```python
from build123d import *

# Parameters (mm, degrees)
F1_DEPTH     = 50.8
F3_DEPTH     = 25.4
F4_T1_DEPTH  = 50.8
F4_T6_DEPTH  = 30.48
F4_S7_R      = 7.62
F4_T8_DEPTH  = 17
F4_T12_DEPTH = 30.48
F4_S13_R     = 7.62
F4_T14_DEPTH = 17
F6_D         = 7.62


# Not quite as in the source:
# - a fillet or chamfer that OpenCascade refuses, or shapes differently, is made with other operations: its cross-section is extruded or revolved along the edge and cut away or added


with BuildPart() as f1:
    # F0 (on Top) → F1 (new body)
    with BuildSketch(Plane.XY):
        with BuildLine():
            Line((0, 25.4), (0, 0))
            Line((0, 0), (50.8, 0))
            Line((50.8, 0), (50.8, 5.08))
            ThreePointArc((50.8, 5.08), (43.18, 12.7), (50.8, 20.32))
            Line((50.8, 20.32), (50.8, 25.4))
            Line((50.8, 25.4), (0, 25.4))
        make_face()
        with BuildLine():
            Line((50.8, 20.32), (50.8, 5.08))
            ThreePointArc((50.8, 5.08), (56.1881536726, 7.3118463274), (58.42, 12.7))
            ThreePointArc((58.42, 12.7), (56.1881536726, 18.0881536726), (50.8, 20.32))
        make_face()
        with BuildLine():
            ThreePointArc((50.8, 20.32), (43.18, 12.7), (50.8, 5.08))
            Line((50.8, 5.08), (50.8, 20.32))
        make_face()
    extrude(amount=F1_DEPTH)

    # F2 (on face) → F3 (cut)
    with BuildSketch(Plane.XZ):
        with BuildLine():
            ThreePointArc((38.1, 25.4), (25.4, 38.1), (12.7, 25.4))
            Line((12.7, 25.4), (38.1, 25.4))
        make_face()
        with BuildLine():
            Line((38.1, 25.4), (12.7, 25.4))
            ThreePointArc((12.7, 25.4), (25.4, 12.7), (38.1, 25.4))
        make_face()
        with BuildLine():
            Line((12.7, 25.4), (12.7, 0))
            Line((12.7, 0), (38.1, 0))
            Line((38.1, 0), (38.1, 25.4))
            ThreePointArc((38.1, 25.4), (25.4, 12.7), (12.7, 25.4))
        make_face()
    extrude(amount=-F3_DEPTH, mode=Mode.SUBTRACT)

    # F4: fillet of radius 5.08 on 3 edges, made by hand

    # F4_s2 → F4_t1 (cut)
    with BuildSketch(Plane.XZ.offset(-38.1)):
        with BuildLine():
            ThreePointArc((0, 45.72), (1.4878975516, 49.3121024484), (5.08, 50.8))
            Line((5.08, 50.8), (0, 50.8))
            Line((0, 50.8), (0, 45.72))
        make_face()
    extrude(amount=F4_T1_DEPTH, mode=Mode.SUBTRACT)


with BuildPart() as f4_tool4:
    # F4_s5 → F4_t6 (new body)
    with BuildSketch(Plane.XZ.offset(12.7)):
        with BuildLine():
            ThreePointArc((45.72, 50.8), (49.3121024484, 49.3121024484), (50.8, 45.72))
            Line((50.8, 45.72), (50.8, 50.8))
            Line((50.8, 50.8), (45.72, 50.8))
        make_face()
    extrude(amount=-F4_T6_DEPTH)

    # F4_s7 → F4_t8 (cut, symmetric)
    with BuildSketch(Plane.XY.offset(48.3)):
        with Locations((50.8, 12.7)):
            Circle(F4_S7_R)
    extrude(amount=F4_T8_DEPTH, both=True, mode=Mode.SUBTRACT)


with BuildPart() as f1_1:
    add(f1.part)

    # F4_t3: cut F4_tool4
    add(f4_tool4.part, mode=Mode.SUBTRACT)


with BuildPart() as f4_tool10:
    # F4_s11 → F4_t12 (new body)
    with BuildSketch(Plane.XZ.offset(-7.62)):
        with BuildLine():
            ThreePointArc((45.72, 50.8), (49.3121024484, 49.3121024484), (50.8, 45.72))
            Line((50.8, 45.72), (50.8, 50.8))
            Line((50.8, 50.8), (45.72, 50.8))
        make_face()
    extrude(amount=-F4_T12_DEPTH)

    # F4_s13 → F4_t14 (cut, symmetric)
    with BuildSketch(Plane.XY.offset(48.3)):
        with Locations((50.8, 12.7)):
            Circle(F4_S13_R)
    extrude(amount=F4_T14_DEPTH, both=True, mode=Mode.SUBTRACT)


with BuildPart() as f1_2:
    add(f1_1.part)

    # F4_t9: cut F4_tool10
    add(f4_tool10.part, mode=Mode.SUBTRACT)

    # F6 (through all)
    with Locations(Plane.XY.offset(50.8)):
        with Locations((50.8, 12.7)):
            Hole(F6_D / 2)


solid = f1_2.part
```
The model under review builds one solid part; all positions refer to its coordinate system, in mm. A direction names the side the tool comes from. Round coordinates to 2 decimals unless told otherwise and drop trailing zeros. Loops run counter-clockwise (first coordinate to the right, second up) from the corner with the lowest first, then second, coordinate; pieces in that order, holes last. Notation, with made-up numbers: M 23,-40 L 54,-40 A25 cw 54,-22 Z; hole C -4,42.25 d10. An arc over 180 degrees is marked long. Answer as a JSON object with one key per item and string values.
(1) Take a section at D-D on z = 46.5. Give the boundary of the cut face in (x, y), and give its area (3 significant figures).
Resolved:
{"outline": "M 0.06,0 L 50.74,0 L 50.74,5.08 A7.62 ccw long 50.74,20.32 L 50.74,25.4 L 0.06,25.4 Z; hole C 50.8,12.7 d7.62", "area": "1,330 mm²"}
(2) Take a section at A-A on y = 22. Give the boundary of the cut face in (x, z).
Resolved:
{"outline": "M 0,0 L 12.7,0 L 12.7,25.4 A12.7 cw 38.1,25.4 L 38.1,0 L 50.8,0 L 50.8,45.72 A5.08 ccw 45.72,50.8 L 5.08,50.8 A5.08 ccw 0,45.72 Z"}
(3) To check wall thickness, follow line 1 along X through (y, z) = (23.75, 6); line 2 along X through (y, z) = (14.75, 9); line 3 along X through (y, z) = (15.25, 28). State the ranges of each line that lie inside material, in increasing order.
Resolved:
{"line 1": "0 to 12.7, 38.1 to 50.8", "line 2": "0 to 12.7, 38.1 to 47.59, 54.01 to 58.14", "line 3": "0 to 12.97, 37.83 to 47.97, 53.63 to 57.98"}
(4) Draft analysis for pull direction X (two halves, no side actions). For faces 6 (the flat face through (50.8, 3, 23)), 7 (the flat face through (46, 13, 0)), 8 (the flat face through (12.7, 13, 13)), state which applies: released by +X, released by -X, zero draft, split by the parting line, or undercut.
Resolved:
{"face 6": "released by +X", "face 7": "zero draft", "face 8": "undercut"}
(5) Take a section at B-B on z = 37. Give the boundary of the cut face in (x, y), and give its area (3 significant figures).
Resolved:
{"outline": "M 0,0 L 20.23,0 L 20.23,25.4 L 0,25.4 Z; M 30.57,0 L 50.8,0 L 50.8,5.08 A7.62 ccw 50.8,20.32 L 50.8,25.4 L 30.57,25.4 Z; hole C 50.8,12.7 d7.62", "area": "1,070 mm²"}
(6) Take a section at C-C on y = 11.75. Give the boundary of the cut face in (x, z).
Resolved:
{"outline": "M 0,0 L 12.7,0 L 12.7,25.4 A12.7 cw 38.1,25.4 L 38.1,0 L 47.11,0 L 47.11,50.8 L 5.08,50.8 A5.08 ccw 0,45.72 Z; M 54.49,0 L 58.36,0 L 58.36,50.8 L 54.49,50.8 Z"}
(7) Tool access review of faces 1 (the cylindrical face through (49.272, 22.621, 49.351)), 2 (the flat face through (6, 13, 0)), 3 (the flat face through (38.1, 13, 13)), 4 (the flat face through (50.8, 23, 23)), 5 (the cylindrical face through (1.449, 12.878, 49.272)): name each direction out of +Z, -Z, +X, -X, +Y, -Y from which nothing blocks a thin tool from reaching the whole face with its end or side.
Resolved:
{"face 1": "+Z, +Y", "face 2": "-Z, +X, -X, +Y, -Y", "face 3": "-Z, +Y, -Y", "face 4": "+Z, -Z, +X, +Y", "face 5": "+Z, -X, +Y, -Y"}
(8) Clearance check with flat-ended pins moving along their axes: P1, Ø1.5, axis at y = 3.5, z = 12.5, coming from the +X side; P2, Ø5, axis at x = 36, y = 8.5, coming from the -Z side; P3, Ø7, axis at x = 50.8, y = 12.7, coming from the -Z side; P4, Ø2, axis at x = 34, y = 21.5, coming from the -Z side. State where each tip first meets the part, or that it passes through.
Resolved:
{"P1": "x = 50.8", "P2": "z = 0", "P3": "through", "P4": "z = 33.71"}
